```python
from build123d import *

# Parameters (mm, degrees)
SKETCH1_W           = 100
SKETCH1_H           = 50
BOSS_EXTRUDE1_DEPTH = 100
SKETCH2_R           = 7.5
CUT_EXTRUDE1_DEPTH  = 151
SKETCH3_W           = 70
SKETCH3_H           = 50
BOSS_EXTRUDE2_DEPTH = 50
SKETCH4_R           = 7.5
CUT_EXTRUDE2_DEPTH  = 135.629120178
SKETCH5_W           = 30
SKETCH5_H           = 20
CUT_EXTRUDE3_DEPTH  = 30
FILLET1_R           = 10


with BuildPart() as part:
    # Sketch1 → Boss-Extrude1 (new body)
    with BuildSketch(Plane(origin=(0, 0, 0), x_dir=(0, 0, -1), z_dir=(1, 0, 0))):
        with Locations((-50, 25)):
            Rectangle(SKETCH1_W, SKETCH1_H)
    extrude(amount=BOSS_EXTRUDE1_DEPTH)

    # Sketch2 → Cut-Extrude1 (cut, through all)
    with BuildSketch(Plane(origin=(0, 0, 0), x_dir=(-1, 0, 0), z_dir=(0, 0, -1))):
        with Locations(Location((-75, 25, 0), (0, 0, 90))):
            Circle(SKETCH2_R)
        with Locations(Location((-25, 25, 0), (0, 0, 90))):
            Circle(SKETCH2_R)
    extrude(amount=-CUT_EXTRUDE1_DEPTH, mode=Mode.SUBTRACT)

    # Sketch3 → Boss-Extrude2 (add)
    with BuildSketch(Plane.XZ):
        with Locations((65, 50)):
            Rectangle(SKETCH3_W, SKETCH3_H)
    extrude(amount=BOSS_EXTRUDE2_DEPTH)

    # Sketch4 → Cut-Extrude2 (cut, through all)
    with BuildSketch(Plane.XY.offset(75)):
        with Locations((85, -35)):
            Circle(SKETCH4_R)
    extrude(amount=-CUT_EXTRUDE2_DEPTH, mode=Mode.SUBTRACT)

    # Sketch5 → Cut-Extrude3 (cut)
    with BuildSketch(Plane.XZ.offset(50)):
        with Locations((85, 50)):
            Rectangle(SKETCH5_W, SKETCH5_H)
    extrude(amount=-CUT_EXTRUDE3_DEPTH, mode=Mode.SUBTRACT)

    # Fillet1
    fillet1_edges = [part.edges().sort_by_distance(p)[0] for p in [
        (100, -50, 32.5),
        (100, -50, 67.5),
        (70, -20, 50),
    ]]
    fillet(fillet1_edges, radius=FILLET1_R)


solid = part.part
```
CAD build for the part. Positions are in the model's coordinates, mm. A direction names the side the tool comes from. Give positions to 0.01 mm unless a question says otherwise; leave off trailing zeros. Order: outer loops, then holes, each group sorted by start corner. A loop starts at its lowest first (then second) coordinate and runs counter-clockwise, first axis right, second up.
(1) Mould opens along Y. For faces 4 (the flat face through (78, -39, 40)), 5 (the cylindrical face through (79.048, -39.564, 32.605)), 6 (the cylindrical face through (97.15, -46.99, 32.61)), 7 (the cylindrical face through (30.1, 19.5, 49.3)) say: released by +Y, released by -Y, zero draft, split by the parting line, or undercut.
(2) Saw through at D-D, the plane x = 62. Give the cut face in (y, z).
(3) Flat gauge pins, fed straight in: pin 1 (24 mm diameter, centred on x = 79.5, y = -33, fed in from +Z); pin 2 (9 mm diameter, centred on x = 81.5, y = -38.5, fed in from -Z); pin 3 (15 mm diameter, centred on y = -19, z = 53.5, fed in from -X). Where does each tip first touch, or does it go through?
(4) Saw through at B-B, the plane y = 25. Give the cut face in (x, z), then the cut area to 3 significant figures.
(5) Saw through at A-A, the plane x = 85. Give the cut face in (y, z).
(6) Tool access for faces 1 (the flat face through (27, 0, 51)), 2 (the flat face through (70, -40, 50)), 3 (the flat face through (65, -25, 75)): list every direction of +Z, -Z, +X, -X, +Y, -Y with a clear straight run to the whole face (end or side of a thin tool).
(7) Saw through at C-C, the plane z = 71. Give the cut face in (x, y), then the cut area to 3 significant figures.
(8) Drill centre lines: L1, parallel to X at y = 25, z = 66; L2, parallel to Y at x = 85, z = 36; L3, parallel to Z at x = 53, y = -5.5. Where is each one in solid material? Low to high.
Results found:
1. face 4: zero draft
1. face 5: undercut
1. face 6: released by -Y
1. face 7: undercut
2. outline: (-50, 25) - (0, 25) - (0, 0) - (50, 0) - (50, 100) - (0, 100) - (0, 75) - (-50, 75) - close
3. pin 1: stops at z = 75
3. pin 2: stops at z = 25
3. pin 3: stops at x = 30
4. outline: (0, 0) - (17.5, 0) - (17.5, 100) - (0, 100) - close; (32.5, 0) - (67.5, 0) - (67.5, 100) - (32.5, 100) - close; (82.5, 0) - (100, 0) - (100, 100) - (82.5, 100) - close
4. area: 7,000 mm2
5. outline: (-50, 25) - (-42.5, 25) - (-42.5, 40) - (-50, 40) - close; (-50, 60) - (-42.5, 60) - (-42.5, 75) - (-50, 75) - close; (-27.5, 25) - (0, 25) - (0, 0) - (50, 0) - (50, 100) - (0, 100) - (0, 75) - (-27.5, 75) - (-27.5, 60) - (-20, 60) - (-20, 40) - (-27.5, 40) - close
6. face 1: -X, -Y
6. face 2: +X, -Y
6. face 3: +Z, +X, -X, -Y
7. outline: (0, 0) - (30, 0) - (30, -50) - (90, -50) arc R10 ccw to (100, -40) - (100, 50) - (0, 50) - close; hole circle Ø15 at (25, 25); hole circle Ø15 at (75, 25); hole circle Ø15 at (85, -35)
7. area: 7,950 mm2
8. L1: x = 0 to 17.5, 32.5 to 67.5, 82.5 to 100
8. L2: y = -50 to -42.5, -27.5 to 50
8. L3: z = 25 to 75
